Input: dimensioned drawing with shaded views. Units: mm. Origin: part minimum x, y, z. Coordinates: 2 decimals unless noted, no trailing zeros. Write each loop counter-clockwise with the first axis right and the second up, starting at its lowest first coordinate (ties: lowest second). Pieces come first, ordered by that corner, then holes. Notation, with made-up numbers: (5.5, 26) - (14.5, 26) arc R25 cw to (14.5, 55) - close; hole circle Ø5 at (-20, 76). An arc over 180 degrees is marked (long way). One line per question, with ' | ' between items.
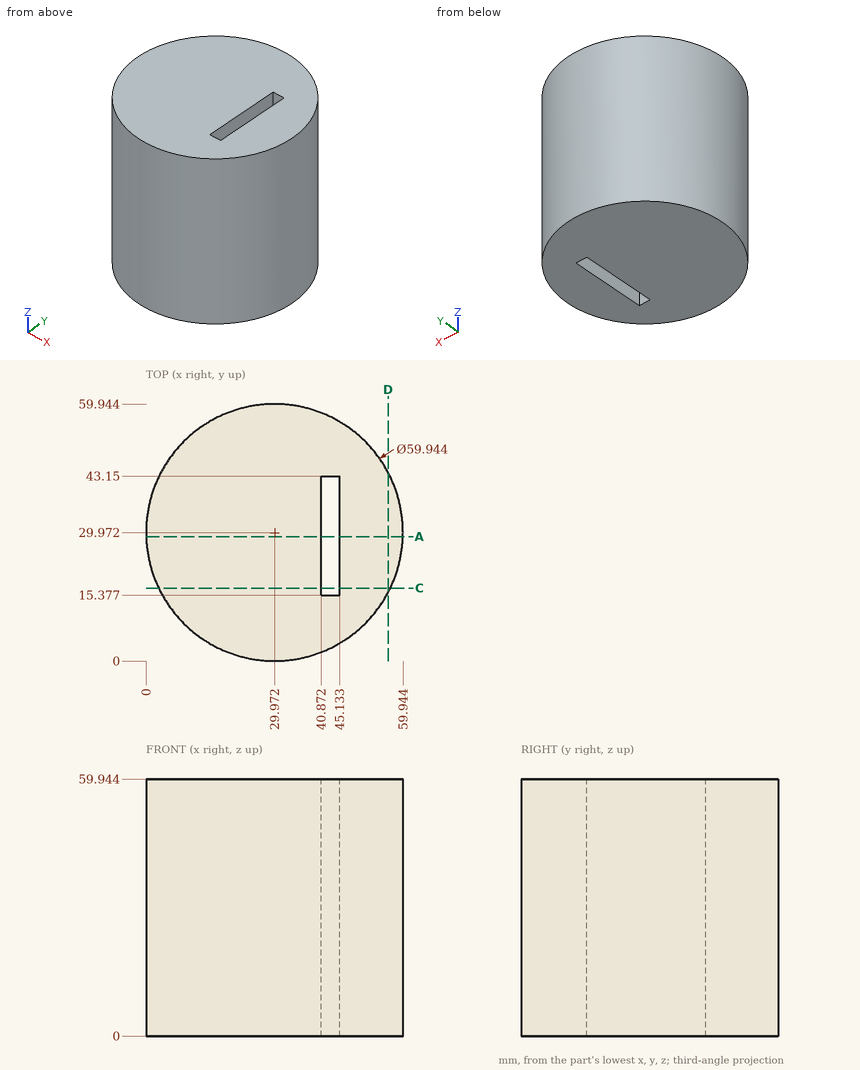
Item 1: Cut plane C-C on y = 17. Return loops of the section in (x, z) (1 decimal).
Check sheet entries:
outline: (3, 0) - (40.9, 0) - (40.9, 59.9) - (3, 59.9) - close; (45.1, 0) - (57, 0) - (57, 59.9) - (45.1, 59.9) - close
Item 2: Ray query, line 1 along X through (y, z) = (30.5, 8) (1 decimal); line 2 along X through (y, z) = (33.5, 52.5) (1 decimal); line 3 along Y through (x, z) = (23.5, 32.5). Return the intervals inside material, ascending. Write a range as [from, to].
Check sheet entries:
line 1: [0, 40.9], [45.1, 59.9] | line 2: [0.2, 40.9], [45.1, 59.7] | line 3: [0.71, 59.24]
Item 3: Cut plane A-A on y = 29. Return loops of the section in (x, z) (1 decimal).
Check sheet entries:
outline: (0, 0) - (40.9, 0) - (40.9, 59.9) - (0, 59.9) - close; (45.1, 0) - (59.9, 0) - (59.9, 59.9) - (45.1, 59.9) - close
Item 4: Cut plane D-D on x = 56.5. Return loops of the section in (y, z) (1 decimal), and give its area (3 significant figures).
Check sheet entries:
outline: (16, 0) - (43.9, 0) - (43.9, 59.9) - (16, 59.9) - close | area: 1,670 mm²
Item 5: Pin query (flat end, axial travel): pin 1 Ø22 at (y, z) = (24, 40) entering from +X; pin 2 Ø8 at (y, z) = (42.5, 20.5) entering from -X; pin 3 Ø4 at (y, z) = (23.5, 23.5) entering from -X (1 decimal); pin 4 Ø3.5 at (x, z) = (43, 44.5) entering from -Y. Return the tip coordinate at first contact, or that it passes through.
Check sheet entries:
pin 1: x = 59.94 | pin 2: x = 1.24 | pin 3: x = 0.3 | pin 4: y = 2.2
